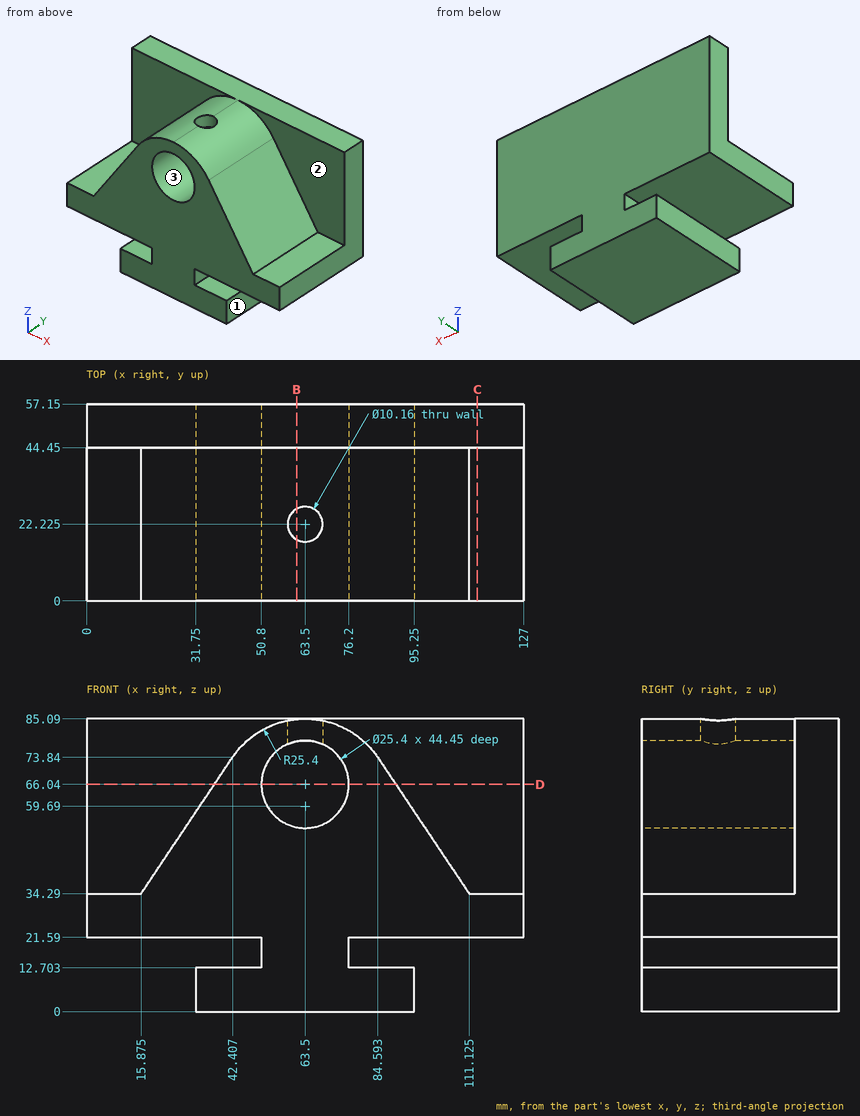
Check sheet for the drawn part. Datum: minimum x, y, z corner. Units: mm. A direction names the side the tool comes from. Give positions to 0.01 mm unless a question says otherwise; leave off trailing zeros. Write each loop counter-clockwise with the first axis right and the second up, starting at its lowest first coordinate (ties: lowest second). Pieces come first, ordered by that corner, then holes. Notation, with made-up numbers: M 35,9 L 83,9 A20 cw 83,36 Z; hole C -8,9.5 d9. An arc over 180 degrees is marked long. One line per question, with ' | ' between items.
1. Cross-section at C-C (x = 113.5). Enter the section's corners in (y, z), plus the area to 3 significant figures.
Ans:
outline: M 0,21.59 L 57.15,21.59 L 57.15,85.09 L 44.45,85.09 L 44.45,34.29 L 0,34.29 Z | area: 1,370 mm2
2. Gauge pin test, flat ends, axial feed: pin 1 (5 mm diameter, centred on x = 98.5, y = 17.5, fed in from +Z) (1 decimal); pin 2 (8 mm diameter, centred on x = 118, y = 15, fed in from +Z); pin 3 (4 mm diameter, centred on y = 42, z = 7, fed in from +X). Record the tip position at first contact, or that the pin passes through.
Ans:
pin 1: z = 56.8 | pin 2: z = 34.29 | pin 3: x = 95.25
3. Set-up check for the marked faces 1, 2 and 3: record each of +Z, -Z, +X, -X, +Y, -Y from which the full face is reachable in a straight line by a thin tool's end or side.
Ans:
face 1: -Z, +X, +Y, -Y | face 2: +Z, +X, -Y | face 3: -Y
4. Cross-section at B-B (x = 61). Enter the section's corners in (y, z).
Ans:
outline: M 0,0 L 57.15,0 L 57.15,85.09 L 44.45,85.09 L 44.45,84.97 L 26.65,84.97 L 26.65,78.49 L 44.45,78.49 L 44.45,53.59 L 0,53.59 Z; M 0,78.49 L 17.8,78.49 L 17.8,84.97 L 0,84.97 Z
5. Scan lines: line 1 along Z through (x, y) = (63.5, 34.5); line 2 along Z through (x, y) = (38, 53); line 3 along Z through (x, y) = (102, 52). Record each from-to range of solid material in increasing order. Write a range as from..to.
Ans:
line 1: 0..53.34, 78.74..85.09 | line 2: 0..12.7, 21.59..85.09 | line 3: 21.59..85.09
6. Cross-section at D-D (z = 66.04). Enter the section's corners in (x, y).
Ans:
outline: M 0,44.45 L 37.17,44.45 L 37.17,0 L 50.8,0 L 50.8,44.45 L 76.2,44.45 L 76.2,0 L 89.83,0 L 89.83,44.45 L 127,44.45 L 127,57.15 L 0,57.15 Z
